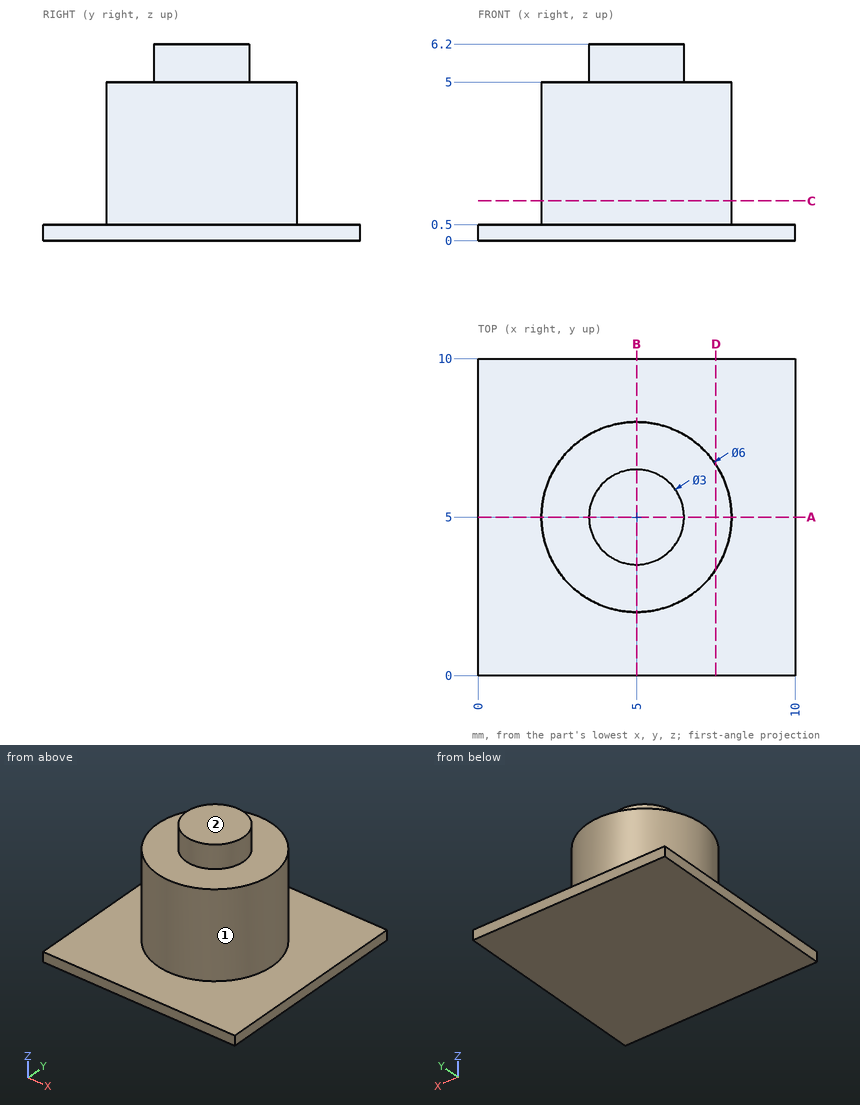
Source: three-view drawing plus pictorial views. Frame: mm from the lowest corner of the part. A direction names the side the tool comes from. Coordinates: 2 decimals unless noted, no trailing zeros. Loops run counter-clockwise (first coordinate to the right, second up) from the corner with the lowest first, then second, coordinate; pieces in that order, holes last. Notation, with made-up numbers: (-19, 25.5) -> (-5, 25.5) arc R17 ccw to (-5, 57.5) -> close; hole circle Ø7 at (25.25, 60.25). An arc over 180 degrees is marked (long way). Write each question's results on one line, items separated by ' | '. Start each with the question number.
Q1. Section D-D, the plane x = 7.5. Return the cut outline in (y, z), plus the area to 3 significant figures.
Q2. Ray query, line 1 (Z direction, x = 4.5, y = 0.75); line 2 (Z direction, x = 3.25, y = 3.25); line 3 (X direction, y = 5, z = 1). Return the intervals inside material, ascending. Write a range as from..to.
Q3. Reachability of the marked faces 1 and 2 from +Z, -Z, +X, -X, +Y, -Y: full face, straight path, thin tool, end or side. Return the list, or none.
Q4. Section C-C, the plane z = 1.25. Return the cut outline in (x, y), plus the area to 3 significant figures.
Q5. Section A-A, the plane y = 5. Return the cut outline in (x, z).
Q6. Pin query (flat end, axial travel): pin 1 (1 mm diameter, centred on y = 5, z = 4, fed in from -X); pin 2 (1 mm diameter, centred on x = 6.5, z = 3.5, fed in from -Y); pin 3 (2 mm diameter, centred on y = 3, z = 4, fed in from -X). Return the tip coordinate at first contact, or that it passes through.
Found:
1) outline: (0, 0) -> (10, 0) -> (10, 0.5) -> (6.66, 0.5) -> (6.66, 5) -> (3.34, 5) -> (3.34, 0.5) -> (0, 0.5) -> close | area: 19.9 mm2
2) line 1: 0..0.5 | line 2: 0..5 | line 3: 2..8
3) face 1: +Z | face 2: +Z, +X, -X, +Y, -Y
4) outline: circle Ø6 at (5, 5) | area: 28.3 mm2
5) outline: (0, 0) -> (10, 0) -> (10, 0.5) -> (8, 0.5) -> (8, 5) -> (6.5, 5) -> (6.5, 6.2) -> (3.5, 6.2) -> (3.5, 5) -> (2, 5) -> (2, 0.5) -> (0, 0.5) -> close
6) pin 1: x = 2 | pin 2: y = 2.17 | pin 3: x = 2.17
